The drawing under review shows one solid part. Ordinate dimensions are in mm from its lowest x, y, z. Coordinates: 2 decimals unless noted, no trailing zeros. Write each loop counter-clockwise with the first axis right and the second up, starting at its lowest first coordinate (ties: lowest second). Pieces come first, ordered by that corner, then holes.
1) Insertion check: P1, Ø1.8, axis at x = 22.5, y = 89.5, coming from the +Z side; P2, Ø5, axis at x = 23, z = 75, coming from the -Y side. Each pin has a flat end and moves straight along its axis. Give the tip position at first contact, or say it passes through.
2) We need section A-A on x = 22.5. Write out the cut boundary in (y, z) (1 decimal).
3) To check wall thickness, follow line 1 along Z through (x, y) = (24, 87.5) (1 decimal); line 2 along X through (y, z) = (116.5, 63.5); line 3 along Z through (x, y) = (20, 71) (1 decimal). State the ranges of each line that lie inside material, in increasing order.
4) We need section B-B on x = 41.5. Write out the cut boundary in (y, z) (1 decimal).
5) Mouldability with a two-part tool opening along X and no side actions: class the marked faces 1, 2 and 3 as pulls with the +X half, pulls with the -X half, needs draft (parallel to the pull), parting line crosses it, or undercut.
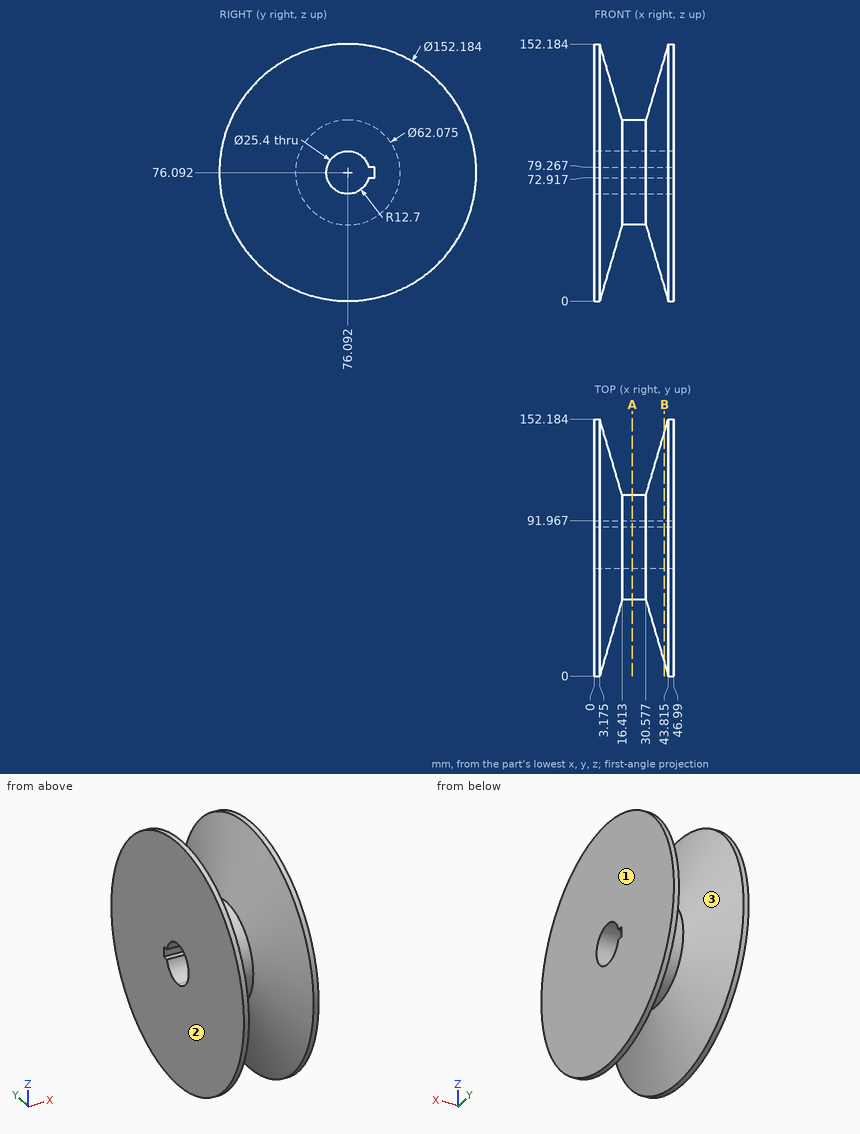
Result:
1. P1: stops at z = 104.5
1. P2: stops at y = 45.05
2. outline: circle Ø62.1 at (76.1, 76.1); hole (88.4, 72.9) - (92, 72.9) - (92, 79.3) - (88.4, 79.3) arc R12.7 ccw (long way) to start
3. line 1: z = 47.2 to 70.5, 81.7 to 105
3. line 2: x = 0 to 13.1, 33.89 to 46.99
3. line 3: z = 45.5 to 64.5, 87.7 to 106.7
4. outline: circle Ø136.4 at (76.1, 76.1); hole (88.4, 72.9) - (92, 72.9) - (92, 79.3) - (88.4, 79.3) arc R12.7 ccw (long way) to start
5. face 1: pulls with the +X half
5. face 2: pulls with the -X half
5. face 3: undercut
